CAD build for the part. Positions are in the model's coordinates, mm. A direction names the side the tool comes from. Coordinates: 2 decimals unless noted, no trailing zeros. Loops run counter-clockwise (first coordinate to the right, second up) from the corner with the lowest first, then second, coordinate; pieces in that order, holes last. Notation, with made-up numbers: (-16, 6) -> (22, 6) arc R24 ccw to (22, 25) -> close; hole circle Ø7 at (-16.5, -28). An arc over 180 degrees is marked (long way). Write each question's results on one line, items separated by ' | '.
from build123d import *

# Parameters (mm, degrees)
F1_DEPTH      = 32
F3_DEPTH      = 1
F3_DEPTH_BACK = 4
F4_R          = 0.4


with BuildPart() as f1:
    # F0 (on Front) → F1 (new body)
    with BuildSketch(Plane.XZ):
        Polygon((0, 128), (0, 0), (25, 0), (25, 135), (20, 147.812783), (-5, 150), (-3.250227, 130), align=None)
    extrude(amount=F1_DEPTH)

    # F2 (on face) → F3 (join, two sides)
    with BuildSketch(Plane(origin=(0, 0, 0), x_dir=(-1, 0, 0), z_dir=(0, 1, 0))) as f3_sk:
        Polygon((4.450136, 139), (5.5, 151), (-6.5, 149.950136), (-7.549864, 137.950136), align=None)
    extrude(amount=F3_DEPTH)
    extrude(f3_sk.sketch, amount=-F3_DEPTH_BACK)

    # F4
    f4_edges = [f1.edges().sort_by_distance(p)[0] for p in [
        (-5.5, -1.5, 151),
        (6.5, -1.5, 149.950136),
        (-4.450136, -1.5, 139),
        (7.549864, 0.5, 137.950136),
    ]]
    fillet(f4_edges, radius=F4_R)


solid = f1.part
1) Slice it at B-B (z = 89). Write the cut outline in (x, y), then the cut area to 3 significant figures.
Outcome:
outline: (0, -32) -> (25, -32) -> (25, 0) -> (0, 0) -> close | area: 800 mm^2
2) Drill centre lines: L1, parallel to Y at x = 10, z = 53; L2, parallel to X at y = -7.5, z = 30.5; L3, parallel to Z at x = 12, y = -10. Where is each one in solid material? Low to high. Write a range as from..to.
Outcome:
L1: y = -32..0 | L2: x = 0..25 | L3: z = 0..148.51
3) Slice it at A-A (y = -18). Write the cut outline in (x, z), then the cut area to 3 significant figures.
Outcome:
outline: (-5, 150) -> (-3.25, 130) -> (0, 128) -> (0, 0) -> (25, 0) -> (25, 135) -> (20, 147.81) -> close | area: 3,770 mm^2
4) Slice it at C-C (x = 9). Write the cut outline in (y, z), then the cut area to 3 significant figures.
Outcome:
outline: (-32, 0) -> (0, 0) -> (0, 148.78) -> (-32, 148.78) -> close | area: 4,760 mm^2
5) Which spindle directions (+Z, -Z, +X, -X, +Y, -Y) get a long thin tool onto all of the face, cutting with end or side? Do faces 1 (the flat face through (6.908, 0.178, 145.29)), 2 (the flat face through (0, -16, 65)), 3 (the flat face through (-4.137, -15.776, 140.14)). Say none if no direction does.
Outcome:
face 1: +Z, +X, +Y | face 2: -Z, -X, +Y, -Y | face 3: -Z, -X, -Y
6) Pin check, flat tips, straight feed: pin 1 (1.5 mm diameter, centred on x = 4, z = 107.5, fed in from +Y); pin 2 (8 mm diameter, centred on y = -18, z = 35.5, fed in from -X). Stop position of each tip, or through.
Outcome:
pin 1: stops at y = 0 | pin 2: stops at x = 0
